Input: part model. Units: mm. Frame: model coordinates. Coordinates: 2 decimals unless noted, no trailing zeros. Write each loop counter-clockwise with the first axis right and the second up, starting at its lowest first coordinate (ties: lowest second). Pieces come first, ordered by that corner, then holes.
from build123d import *

# Parameters (mm, degrees)
SKETCH1_W           = 160
SKETCH1_H           = 50
BOSS_EXTRUDE1_DEPTH = 1.25
SKETCH2_W           = 10
SKETCH2_H           = 2.5
SKETCH2_W_2         = 15
CUT_EXTRUDE1_DEPTH  = 4
SKETCH3_W           = 2.5
SKETCH3_H           = 22.5
CUT_EXTRUDE2_DEPTH  = 84.852549156


with BuildPart() as part:
    # Sketch1 → Boss-Extrude1 (new, symmetric)
    with BuildSketch(Plane(origin=(0, 0, 0), x_dir=(1, 0, 0), z_dir=(0, 1, 0))):
        Rectangle(SKETCH1_W, SKETCH1_H)
    extrude(amount=BOSS_EXTRUDE1_DEPTH, both=True)

    # Sketch2 → Cut-Extrude1 (cut)
    with BuildSketch(Plane(origin=(0, 1.25, 0), x_dir=(1, 0, 0), z_dir=(0, 1, 0))):
        with Locations((30, 23.75)):
            Rectangle(SKETCH2_W, SKETCH2_H)
        with Locations((10, 23.75)):
            Rectangle(SKETCH2_W, SKETCH2_H)
        with Locations((10, -23.75)):
            Rectangle(SKETCH2_W, SKETCH2_H)
        with Locations((30, -23.75)):
            Rectangle(SKETCH2_W, SKETCH2_H)
        with Locations((50, 23.75)):
            Rectangle(SKETCH2_W, SKETCH2_H)
        with Locations((50, -23.75)):
            Rectangle(SKETCH2_W, SKETCH2_H)
        with Locations((-10, 23.75)):
            Rectangle(SKETCH2_W, SKETCH2_H)
        with Locations((-10, -23.75)):
            Rectangle(SKETCH2_W, SKETCH2_H)
        with Locations((-30, 23.75)):
            Rectangle(SKETCH2_W, SKETCH2_H)
        with Locations((-30, -23.75)):
            Rectangle(SKETCH2_W, SKETCH2_H)
        with Locations((-50, 23.75)):
            Rectangle(SKETCH2_W, SKETCH2_H)
        with Locations((-50, -23.75)):
            Rectangle(SKETCH2_W, SKETCH2_H)
        with Locations((72.5, 23.75)):
            Rectangle(SKETCH2_W_2, SKETCH2_H)
        with Locations((72.5, -23.75)):
            Rectangle(SKETCH2_W_2, SKETCH2_H)
        with Locations((-72.5, 23.75)):
            Rectangle(SKETCH2_W_2, SKETCH2_H)
        with Locations((-72.5, -23.75)):
            Rectangle(SKETCH2_W_2, SKETCH2_H)
    extrude(amount=-CUT_EXTRUDE1_DEPTH, mode=Mode.SUBTRACT)

    # Sketch3 → Cut-Extrude2 (cut, through all)
    with BuildSketch(Plane(origin=(0, 1.25, 0), x_dir=(1, 0, 0), z_dir=(0, 1, 0))):
        with Locations((78.75, -11.25)):
            Rectangle(SKETCH3_W, SKETCH3_H)
        with Locations((-78.75, -11.25)):
            Rectangle(SKETCH3_W, SKETCH3_H)
    extrude(amount=-CUT_EXTRUDE2_DEPTH, mode=Mode.SUBTRACT)


solid = part.part
Item 1: Section query B-B, the plane x = 11. Return loops of the section in (y, z), then the cut area to 4 significant figures.
Item 2: Pin query (flat end, axial travel): pin 1 Ø1.2 at (y, z) = (-0.5, -23.5) entering from +X; pin 2 Ø1.2 at (x, y) = (-48, 0.5) entering from +Z; pin 3 Ø1.2 at (y, z) = (0.5, 23) entering from +X. Return the tip coordinate at first contact, or that it passes through.
Item 3: Section query A-A, the plane z = 21. Return loops of the section in (x, y).
Item 4: Material intervals for line 1 (X direction, y = -0.3, z = 19.5); line 2 (Z direction, x = 5.5, y = -0.5), sorted ascending.
The answers:
1. outline: (-1.25, -22.5) - (1.25, -22.5) - (1.25, 22.5) - (-1.25, 22.5) - close
1. area: 112.5 mm2
2. pin 1: stops at x = 65
2. pin 2: stops at z = 22.5
2. pin 3: stops at x = 77.5
3. outline: (-77.5, -1.25) - (77.5, -1.25) - (77.5, 1.25) - (-77.5, 1.25) - close
4. line 1: x = -77.5 to 77.5
4. line 2: z = -22.5 to 22.5
